Here's how the part is built. I have some questions about the finished solid (model axes, mm). A direction names the side the tool comes from. Round coordinates to 2 decimals unless told otherwise and drop trailing zeros. Loops run counter-clockwise (first coordinate to the right, second up) from the corner with the lowest first, then second, coordinate; pieces in that order, holes last. Notation, with made-up numbers: M -27.5,40.5 L -14.5,40.5 A9 ccw -14.5,49.5 Z; hole C -37.5,13.5 d8. An arc over 180 degrees is marked long. Answer as a JSON object with one key per item and string values.
from build123d import *

# Parameters (mm, degrees)
SKETCH1_W           = 10
SKETCH1_H           = 10
SKETCH1_W_2         = 8
SKETCH1_H_2         = 8
BOSS_EXTRUDE1_DEPTH = 60
SKETCH2_R           = 2.025
CUT_EXTRUDE1_DEPTH  = 62.032778079
SKETCH4_R           = 2.025
CUT_EXTRUDE2_DEPTH  = 62.032778079


with BuildPart() as part:
    # Sketch1 → Boss-Extrude1 (new body)
    with BuildSketch(Plane(origin=(0, 0, 0), x_dir=(1, 0, 0), z_dir=(0, 1, 0))):
        Rectangle(SKETCH1_W, SKETCH1_H)
        Rectangle(SKETCH1_W_2, SKETCH1_H_2, mode=Mode.SUBTRACT)
    extrude(amount=BOSS_EXTRUDE1_DEPTH)

    # Sketch2 → Cut-Extrude1 (cut, through all)
    with BuildSketch(Plane(origin=(5, 0, 0), x_dir=(0, 0, -1), z_dir=(1, 0, 0))):
        with Locations((0, 5)):
            Circle(SKETCH2_R)
        with Locations((0, 25)):
            Circle(SKETCH2_R)
    extrude(amount=-CUT_EXTRUDE1_DEPTH, mode=Mode.SUBTRACT)

    # Sketch4 → Cut-Extrude2 (cut, through all)
    with BuildSketch(Plane.XY.offset(5)):
        with Locations((0, 55)):
            Circle(SKETCH4_R)
        with Locations((0, 40)):
            Circle(SKETCH4_R)
    extrude(amount=-CUT_EXTRUDE2_DEPTH, mode=Mode.SUBTRACT)


solid = part.part
Item 1: For P1, Ø3.5, axis at x = 0, y = 40, coming from the +Z side, with a flat end and sliding along its axis, tell me the tip position at first contact or that it passes through.
Solution:
{"P1": "passes through"}
Item 2: I want a section at A-A on x = 2.75. List the corners of the cut face in (y, z) for me.
Solution:
{"outline": "M 0,-5 L 60,-5 L 60,-4 L 0,-4 Z; M 0,4 L 60,4 L 60,5 L 0,5 Z"}
Item 3: For faces 1 (the face through (-4.5, 0, -0.1)), 2 (the face through (4, 30, 0)), which set-ups out of +Z, -Z, +X, -X, +Y, -Y let a thin tool reach every point of the face, with its end or its side?
Solution:
{"face 1": "+Z, -Z, +X, -X, -Y", "face 2": "+Y, -Y"}
Item 4: I want a section at B-B on z = 2.75. List the corners of the cut face in (x, y) for me.
Solution:
{"outline": "M -5,0 L -4,0 L -4,60 L -5,60 Z; M 4,0 L 5,0 L 5,60 L 4,60 Z"}
Item 5: If I drill on L1, parallel to Y at x = -4.6, z = 0 (3 decimals); L2, parallel to Z at x = 2.25, y = 37, over which ranges is the centre line in solid material (lowest first)? Write a range as from..to.
Solution:
{"L1": "y = 0..2.975, 7.025..22.975, 27.025..60", "L2": "z = -5..-4, 4..5"}
Item 6: I want a section at D-D on x = -0.75. List the corners of the cut face in (y, z) for me, plus the area to 3 significant figures.
Solution:
{"outline": "M 0,-5 L 38.12,-5 L 38.12,-4 L 0,-4 Z; M 0,4 L 38.12,4 L 38.12,5 L 0,5 Z; M 41.88,-5 L 53.12,-5 L 53.12,-4 L 41.88,-4 Z; M 41.88,4 L 53.12,4 L 53.12,5 L 41.88,5 Z; M 56.88,-5 L 60,-5 L 60,-4 L 56.88,-4 Z; M 56.88,4 L 60,4 L 60,5 L 56.88,5 Z", "area": "105 mm2"}
Item 7: I want a section at C-C on y = 8.5. List the corners of the cut face in (x, z) for me.
Solution:
{"outline": "M -5,-5 L 5,-5 L 5,5 L -5,5 Z; hole M -4,-4 L 4,-4 L 4,4 L -4,4 Z"}
Item 8: We'd pull the mould along X, two halves only. Please class faces 3 (the face through (1.1, 41.7, -4.5)), 4 (the face through (5, 30, 0)), 5 (the face through (-5, 30, 0)): +X half, -X half, draft (parallel to the pull), parting line (faces both ways), or undercut.
Solution:
{"face 3": "undercut", "face 4": "+X half", "face 5": "-X half"}
